Work out the finished part from the listing and answer in its coordinate system (mm). Face numbers are marked on the shaded views. A direction names the side the tool comes from. Coordinates: 2 decimals unless noted, no trailing zeros. Write each loop counter-clockwise with the first axis right and the second up, starting at its lowest first coordinate (ties: lowest second). Pieces come first, ordered by that corner, then holes. Notation, with made-up numbers: (-13.75, -30.75) - (45.25, -30.75) arc R24 ccw to (45.25, -19.75) - close; hole circle Ø1 at (42.5, 12.25). An arc over 180 degrees is marked (long way). One line per item, written item: value.
```python
from build123d import *

# Parameters (mm, degrees)
F0_W     = 270
F0_H     = 15
F0_W_2   = 235
F0_W_3   = 15
F0_H_2   = 185
F0_H_3   = 170
F1_DEPTH = 300
F2_R     = 100
F3_DEPTH = 15
F4_R     = 89.325902


with BuildPart() as f1:
    # F0 (on Front) → F1 (new body)
    with BuildSketch(Plane.XZ):
        with Locations((-135, 192.5)):
            Rectangle(F0_W, F0_H)
        with Locations((132.5, 7.5)):
            Rectangle(F0_W_2, F0_H)
        with Locations((-277.5, 92.5)):
            Rectangle(F0_W_3, F0_H_2)
        with Locations((7.5, 7.5)):
            Rectangle(F0_W_3, F0_H)
        with Locations((7.5, 100)):
            Rectangle(F0_W_3, F0_H_3)
        with Locations((7.5, 192.5)):
            Rectangle(F0_W_3, F0_H)
        with Locations((-277.5, 192.5)):
            Rectangle(F0_W_3, F0_H)
    extrude(amount=-F1_DEPTH)

    # F2 (on face) → F3 (cut, through all)
    with BuildSketch(Plane.XY.offset(200)):
        with Locations((-135, 150)):
            Circle(F2_R)
    extrude(amount=-F3_DEPTH, mode=Mode.SUBTRACT)

    # F4
    f4_edges = [f1.edges().sort_by_distance(p)[0] for p in [
        (15, 150, 15),
        (0, 150, 0),
    ]]
    fillet(f4_edges, radius=F4_R)


solid = f1.part
```
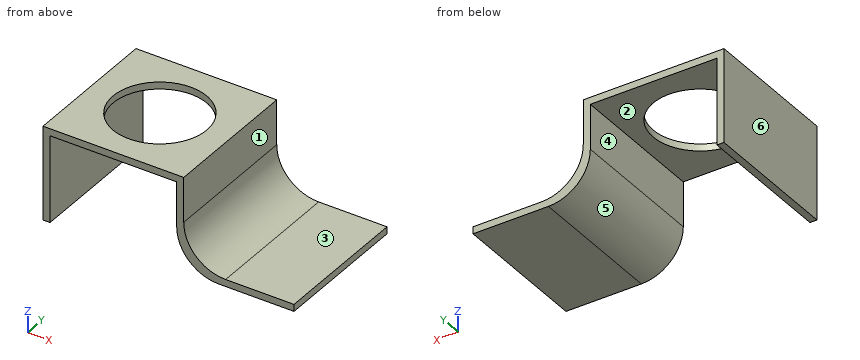
Item 1: Which of the six approach directions +Z, -Z, +X, -X, +Y, -Y give full straight-line access (tool end or side, diameter ignored) to the marked faces 5 and 6?
Evaluation:
face 5: -Z, +Y, -Y
face 6: +Z, -Z, -X, +Y, -Y
Item 2: Section B-B, the plane z = 156 is taken. Determine the outline of the cut face in (x, y).
Evaluation:
outline: (-285, 0) - (-270, 0) - (-270, 300) - (-285, 300) - close; (0, 0) - (15, 0) - (15, 300) - (0, 300) - close
Item 3: Section A-A, the plane x = -135 is taken. Determine the outline of the cut face in (y, z), then the cut area to 3 significant figures.
Evaluation:
outline: (0, 185) - (50, 185) - (50, 200) - (0, 200) - close; (250, 185) - (300, 185) - (300, 200) - (250, 200) - close
area: 1,500 mm2
Item 4: Section C-C, the plane y = 150 is taken. Determine the outline of the cut face in (x, z), then the cut area to 3 significant figures.
Evaluation:
outline: (-285, 0) - (-270, 0) - (-270, 185) - (-235, 185) - (-235, 200) - (-285, 200) - close; (-35, 185) - (0, 185) - (0, 89.33) arc R89.33 ccw to (89.33, 0) - (250, 0) - (250, 15) - (104.33, 15) arc R89.33 cw to (15, 104.33) - (15, 200) - (-35, 200) - close
area: 10,600 mm2
Item 5: Consider probe 1 along Y at (x, z) = (-135, 190.75); probe 2 along Z at (x, y) = (-204.5, 257); probe 3 along Z at (x, y) = (127.5, 178). Determine where each line is inside the solid, lowest interval first.
Evaluation:
probe 1: y = 0 to 50, 250 to 300
probe 2: z = 185 to 200
probe 3: z = 0 to 15
Item 6: Given pin 1 (10 mm diameter, centred on x = -163, y = 243, fed in from -Z); pin 2 (1.5 mm diameter, centred on y = 152, z = 154.5, fed in from +X); pin 3 (12 mm diameter, centred on y = 73.5, z = 87, fed in from +X), each flat-ended and moving along its own axis, determine where each tip first touches the part or whether it passes through.
Evaluation:
pin 1: stops at z = 185
pin 2: stops at x = 15
pin 3: stops at x = 18.1
Item 7: Section D-D, the plane x = 185 is taken. Determine the outline of the cut face in (y, z).
Evaluation:
outline: (0, 0) - (300, 0) - (300, 15) - (0, 15) - close
Item 8: Determine the mould class of the marked faces 1, 2, 3 and 4 for opening direction X: +X half, -X half, draft (parallel to the pull), parting line (faces both ways), or undercut.
Evaluation:
face 1: +X half
face 2: undercut
face 3: draft
face 4: undercut
